Work out the finished part from the listing and answer in its coordinate system (mm). Face numbers are marked on the shaded views. A direction names the side the tool comes from. Coordinates: 2 decimals unless noted, no trailing zeros. Write each loop counter-clockwise with the first axis right and the second up, starting at its lowest first coordinate (ties: lowest second). Pieces come first, ordered by that corner, then holes. Notation, with made-up numbers: (18, -27.5) - (77, -27.5) arc R15 cw to (77, -22.5) - close; hole circle Ø7 at (11.25, 41). An arc over 180 degrees is marked (long way). Use CSV: the item, a comma, the result in double quotes. Start each with the question number.
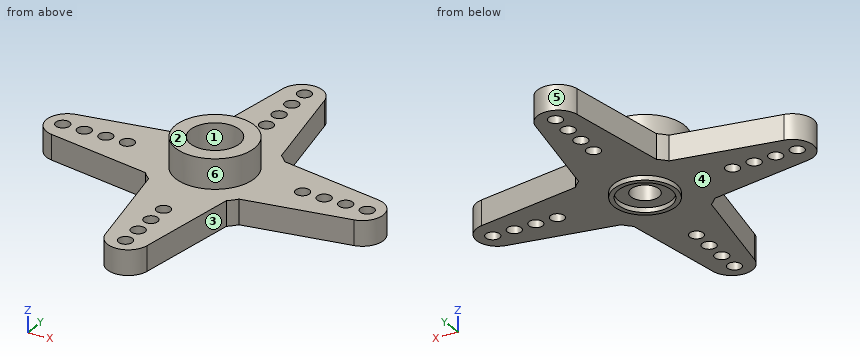
from build123d import *

# Parameters (mm, degrees)
ESBO_O1_R                = 0.75
ESBO_O1_R_2              = 1.5
RESSALTO_EXTRUS_O1_DEPTH = 2.7
PADR_OCIRCULAR1_COUNT    = 4
ESBO_O2_R                = 4.25
ESBO_O2_R_2              = 2.65
RESSALTO_EXTRUS_O2_DEPTH = 3.2
ESBO_O3_R                = 3.35
ESBO_O3_R_2              = 2.85
RESSALTO_EXTRUS_O3_DEPTH = 0.5


with BuildPart() as part:
    # Esboço1 → Ressalto-extrusão1 (new body)
    with BuildSketch(Plane.XY):
        with BuildLine():
            Line((-2.21682252, 16.134964821), (-4.15, 5.002749244))
            ThreePointArc((-4.15, 5.002749244), (0, -6.5), (4.15, 5.002749244))
            Line((4.15, 5.002749244), (2.21682252, 16.134964821))
            ThreePointArc((2.21682252, 16.134964821), (0, 18), (-2.21682252, 16.134964821))
        make_face()
        with Locations(Location((0, 16.25, 0), (0, 0, 180))):
            Circle(ESBO_O1_R, mode=Mode.SUBTRACT)
        with Locations(Location((0, 13.95, 0), (0, 0, 180))):
            Circle(ESBO_O1_R, mode=Mode.SUBTRACT)
        with Locations(Location((0, 11.65, 0), (0, 0, 180))):
            Circle(ESBO_O1_R, mode=Mode.SUBTRACT)
        with Locations(Location((0, 9.35, 0), (0, 0, 180))):
            Circle(ESBO_O1_R, mode=Mode.SUBTRACT)
        with Locations(Location((0, 0, 0), (0, 0, 180))):
            Circle(ESBO_O1_R_2, mode=Mode.SUBTRACT)
    ressalto_extrus_o1 = extrude(amount=RESSALTO_EXTRUS_O1_DEPTH)

    # PadrãoCircular1: Ressalto-extrusão1 ×4 about axis
    padr_ocircular1_axis = Axis((0, 0, 0), (0, 0, 1))
    for i in range(1, PADR_OCIRCULAR1_COUNT):
        add(ressalto_extrus_o1.rotate(padr_ocircular1_axis, i * 360 / PADR_OCIRCULAR1_COUNT))

    # Esboço2 → Ressalto-extrusão2 (add)
    with BuildSketch(Plane.XY.offset(2.7)):
        Circle(ESBO_O2_R)
        Circle(ESBO_O2_R_2, mode=Mode.SUBTRACT)
    extrude(amount=RESSALTO_EXTRUS_O2_DEPTH)

    # Esboço3 → Ressalto-extrusão3 (add)
    with BuildSketch(Plane(origin=(0, 0, 0), x_dir=(-1, 0, 0), z_dir=(0, 0, -1))):
        with Locations(Location((0, 0, 0), (0, 0, 180))):
            Circle(ESBO_O3_R)
        Circle(ESBO_O3_R_2, mode=Mode.SUBTRACT)
    extrude(amount=RESSALTO_EXTRUS_O3_DEPTH)


solid = part.part
Item 1: A cutting plane is placed at B-B (x = -11.65). Determine the outline of the cut face in (y, z).
Item 2: Each of these flat-tipped pins is pushed along its axis until it touches: pin 1 (1.7 mm diameter, centred on x = -16.25, y = 0, fed in from -Z); pin 2 (1.5 mm diameter, centred on y = 13, z = 1.5, fed in from -X); pin 3 (4 mm diameter, centred on x = 0, y = -0.5, fed in from +Z); pin 4 (1.5 mm diameter, centred on y = 14, z = 4.5, fed in from -X). Where does it stop, or does it pass through?
Item 3: A cutting plane is placed at A-A (y = 9.35). Determine the outline of the cut face in (x, z), then the cut area to 3 significant figures.
Item 4: Determine the mould class of the marked faces 1, 2 and 3 for opening direction Y: +Y half, -Y half, draft (parallel to the pull), parting line (faces both ways), or undercut.
Item 5: Which of the six approach directions +Z, -Z, +X, -X, +Y, -Y give full straight-line access (tool end or side, diameter ignored) to the marked faces 4, 5 and 6?
Item 6: Straight lines are drawn through the part: probe 1 along Y at (x, z) = (0, -0.3); probe 2 along Y at (x, z) = (-9.5, 1.25); probe 3 along Z at (x, y) = (1.5, -12.5). For each, find the intervals that lie inside material, in ascending order. Write a range as [from, to].
Item 7: A cutting plane is placed at C-C (z = 0.75). Count the separate pieces of the cut face and the enclosed holes in it, then the cut area to 3 significant figures.
Calculated:
1,outline,"(-3, 0) - (-0.75, 0) - (-0.75, 2.7) - (-3, 2.7) - close; (0.75, 0) - (3, 0) - (3, 2.7) - (0.75, 2.7) - close"
2,pin 1,"stops at z = 0"
2,pin 2,"stops at x = -2.89"
2,pin 3,"stops at z = 2.7"
2,pin 4,"passes through"
3,outline,"(-3.4, 0) - (-0.75, 0) - (-0.75, 2.7) - (-3.4, 2.7) - close; (0.75, 0) - (3.4, 0) - (3.4, 2.7) - (0.75, 2.7) - close"
3,area,"14.3 mm²"
4,face 1,"undercut"
4,face 2,"draft"
4,face 3,"-Y half"
5,face 4,"-Z"
5,face 5,"+Z, -Z, +Y"
5,face 6,"+Z"
6,probe 1,"y = [-3.35, -2.85], [2.85, 3.35]"
6,probe 2,"y = [-3.37, -0.73], [0.73, 3.37]"
6,probe 3,"z = [0, 2.7]"
7,separate pieces,"1"
7,enclosed holes,"17"
7,area,"372 mm²"
